from build123d import *

# Parameters (mm, degrees)
SKETCH1_R               = 12.65
BOSS_EXTRUDE1_DEPTH     = 6.35
SKETCH2_R               = 9.6
CUT_EXTRUDE1_DEPTH      = 7.35
CUT_EXTRUDE1_DEPTH_BACK = 7.35
SKETCH3_R               = 10.15238
CUT_EXTRUDE2_DEPTH      = 3
SKETCH4_R               = 10.16
CUT_EXTRUDE3_DEPTH      = 10.826
SKETCH6_R               = 10.66038
CUT_EXTRUDE4_DEPTH      = 1
FILLET1_R               = 0.5


with BuildPart() as part:
    # Sketch1 → Boss-Extrude1 (new body, symmetric)
    with BuildSketch(Plane(origin=(0, 0, 0), x_dir=(1, 0, 0), z_dir=(0, 1, 0))):
        Circle(SKETCH1_R)
    extrude(amount=BOSS_EXTRUDE1_DEPTH, both=True)

    # Sketch2 → Cut-Extrude1 (cut, two sides)
    with BuildSketch(Plane(origin=(0, 0, 0), x_dir=(1, 0, 0), z_dir=(0, 1, 0))) as cut_extrude1_sk:
        Circle(SKETCH2_R)
    extrude(amount=CUT_EXTRUDE1_DEPTH, mode=Mode.SUBTRACT)
    extrude(cut_extrude1_sk.sketch, amount=-CUT_EXTRUDE1_DEPTH_BACK, mode=Mode.SUBTRACT)

    # Sketch3 → Cut-Extrude2 (cut, symmetric)
    with BuildSketch(Plane(origin=(0, 0, 0), x_dir=(1, 0, 0), z_dir=(0, 1, 0))):
        Circle(SKETCH3_R)
    extrude(amount=CUT_EXTRUDE2_DEPTH, both=True, mode=Mode.SUBTRACT)

    # Sketch4 → Cut-Extrude3 (cut)
    with BuildSketch(Plane(origin=(0, 0, 0), x_dir=(1, 0, 0), z_dir=(0, 1, 0))):
        Circle(SKETCH4_R)
    extrude(amount=CUT_EXTRUDE3_DEPTH, mode=Mode.SUBTRACT)

    # Sketch6 → Cut-Extrude4 (cut)
    with BuildSketch(Plane(origin=(0, 2.9972, 0), x_dir=(1, 0, 0), z_dir=(0, 1, 0))):
        Circle(SKETCH6_R)
    extrude(amount=CUT_EXTRUDE4_DEPTH, mode=Mode.SUBTRACT)

    # Fillet1
    fillet1_edges = [part.edges().sort_by_distance(p)[0] for p in [
        (-12.65, -6.35, 0),
        (-12.65, 6.35, 0),
    ]]
    fillet(fillet1_edges, radius=FILLET1_R)


solid = part.part
Can you work these out from the model? Positions are in its coordinate system, mm. A direction names the side the tool comes from. Give positions to 0.01 mm unless a question says otherwise; leave off trailing zeros. Loops run counter-clockwise (first coordinate to the right, second up) from the corner with the lowest first, then second, coordinate; pieces in that order, holes last. Notation, with made-up numbers: (-2, 13.5) - (16, 13.5) arc R19 cw to (16, 23.5) - close; hole circle Ø9 at (19.5, 8.25). An arc over 180 degrees is marked (long way). Return JSON: item names as keys, results as strings.
1. If I drill on line 1 (X direction, y = 1.45, z = 0); line 2 (Z direction, x = 0, y = 3.2); line 3 (Z direction, x = 0, y = -0.6), over which ranges is the centre line in solid material (lowest first)?
Output values:
{"line 1": "x = -12.65 to -10.16, 10.16 to 12.65", "line 2": "z = -12.65 to -10.66, 10.66 to 12.65", "line 3": "z = -12.65 to -10.15, 10.15 to 12.65"}
2. For faces 5 (the face through (-1.323, 1.478, -10.074)), 6 (the face through (-3, 6.35, 10)), which set-ups out of +Z, -Z, +X, -X, +Y, -Y let a thin tool reach every point of the face, with its end or its side?
Output values:
{"face 5": "+Y", "face 6": "+Z, -Z, +X, -X, +Y"}
3. We'd pull the mould along Y, two halves only. Please class faces 1 (the face through (5.161, -4.652, -8.095)), 2 (the face through (4, -3, 9)), 3 (the face through (9, -6.35, -4)), 4 (the face through (10.17, 3.49, -3.2)): +Y half, -Y half, draft (parallel to the pull), parting line (faces both ways), or undercut.
Output values:
{"face 1": "draft", "face 2": "+Y half", "face 3": "-Y half", "face 4": "undercut"}
4. I want a section at C-C on y = -2.5. Please give me the cut outline in (x, z).
Output values:
{"outline": "circle Ø25.3 at (0, 0); hole circle Ø20.3 at (0, 0)"}
5. I'm going to push flat-ended pins straight in: pin 1 Ø2 at (x, y) = (-3, -5) entering from -Z; pin 2 Ø5 at (y, z) = (2, -9) entering from -X; pin 3 Ø1 at (x, y) = (6, -3) entering from +Z. Where does each tip first touch, or does it pass through?
Output values:
{"pin 1": "stops at z = -12.49", "pin 2": "stops at x = -10.85", "pin 3": "stops at z = 11.39"}
